Can you work these out from the model? Positions are in its coordinate system, mm. A direction names the side the tool comes from. Coordinates: 2 decimals unless noted, no trailing zeros. Order: outer loops, then holes, each group sorted by start corner. A loop starts at its lowest first (then second) coordinate and runs counter-clockwise, first axis right, second up. Notation, with made-up numbers: M 70,-11.5 L 84,-11.5 A16 ccw 84,5.5 Z; hole C 48.25,-33 d6. An arc over 180 degrees is marked long. Answer as CSV lines item,"result". Start each with the question number.
1. Will these pins go through, and if not, where does the flat tip stop? pin 1 (10 mm diameter, centred on x = 11, z = 24, fed in from +Y); pin 2 (9 mm diameter, centred on x = 10.5, y = 6, fed in from +Z); pin 3 (8 mm diameter, centred on x = 10, y = 5.5, fed in from -Z).
2. If we section it at A-A (x = 10): List the corners of the cut face in (y, z) for me, plus the area to 3 significant figures.
3. If we section it at C-C (z = 30): List the corners of the cut face in (x, y) for me.
4. I need wall thicknesses on line 1 along X through (y, z) = (-16, 30); line 2 along Y through (x, z) = (10, 2.5); line 3 along Y through (x, z) = (9.5, 39). Which ranges of each line are inside material? Lowest first, please. Write a range as from..to.
5. If we section it at D-D (x = 6.25): List the corners of the cut face in (y, z) for me.
6. If we mould it in two halves opening along Y, with no side actions, what happens to faces 1 (the face through (10, -15, 30)), 2 (the face through (20, -10, 30)), 3 (the face through (14.619, 3.585, 4.93)), 4 (the face through (10.229, 11.496, 4.93))? For each: released by +Y, released by -Y, zero draft, split by the parting line, or undercut.
7. On a 3-axis mill with a long thin cutter (end or side, diameter ignored), from which of +Z, -Z, +X, -X, +Y, -Y can I reach the whole of each face in a straight line? I mean faces 5 (the face through (10, -8, 0)), 6 (the face through (8.6, 10.5, 10)), 7 (the face through (8.418, -17.535, 32.063)). Say none if no direction works.
8. If we section it at B-B (y = 5.5): List the corners of the cut face in (x, z) for me, plus the area to 3 significant figures.
```python
from build123d import *

# Parameters (mm, degrees)
SKETCH1_W           = 20
SKETCH1_H           = 20
BOSS_EXTRUDE1_DEPTH = 60
SKETCH2_R           = 2.6
CUT_EXTRUDE1_DEPTH  = 5
SKETCH3_R           = 6
SKETCH3_R_2         = 5
BOSS_EXTRUDE2_DEPTH = 10


with BuildPart() as part:
    # Sketch1 → Boss-Extrude1 (new body)
    with BuildSketch(Plane.XY):
        with Locations((10, -10)):
            Rectangle(SKETCH1_W, SKETCH1_H)
    extrude(amount=BOSS_EXTRUDE1_DEPTH)

    # Sketch2 → Cut-Extrude1 (cut)
    with BuildSketch(Plane.XZ.offset(20)):
        with Locations(Location((10, 30, 0), (0, 0, 270))):
            Circle(SKETCH2_R)
    extrude(amount=-CUT_EXTRUDE1_DEPTH, mode=Mode.SUBTRACT)

    # Sketch3 → Boss-Extrude2 (add)
    with BuildSketch(Plane.XY):
        with Locations((10, 5.5)):
            Circle(SKETCH3_R)
        with Locations((10, 5.5)):
            Circle(SKETCH3_R_2, mode=Mode.SUBTRACT)
    extrude(amount=BOSS_EXTRUDE2_DEPTH)


solid = part.part
```
Solved:
1,pin 1,"y = 0"
1,pin 2,"z = 10"
1,pin 3,"through"
2,outline,"M -20,0 L 0.5,0 L 0.5,10 L 0,10 L 0,60 L -20,60 L -20,32.6 L -15,32.6 L -15,27.4 L -20,27.4 Z; M 10.5,0 L 11.5,0 L 11.5,10 L 10.5,10 Z"
2,area,"1,190 mm²"
3,outline,"M 0,-20 L 7.4,-20 L 7.4,-15 L 12.6,-15 L 12.6,-20 L 20,-20 L 20,0 L 0,0 Z"
4,line 1,"0..7.4, 12.6..20"
4,line 2,"-20..0.5, 10.5..11.5"
4,line 3,"-20..0"
5,outline,"M -20,0 L 0,0 L 0,60 L -20,60 Z; M 0.82,0 L 2.19,0 L 2.19,10 L 0.82,10 Z; M 8.81,0 L 10.18,0 L 10.18,10 L 8.81,10 Z"
6,face 1,"released by -Y"
6,face 2,"zero draft"
6,face 3,"undercut"
6,face 4,"undercut"
7,face 5,"-Z, +X, -X, +Y, -Y"
7,face 6,"+Z, +X, -X, +Y"
7,face 7,"-Y"
8,outline,"M 4,0 L 5,0 L 5,10 L 4,10 Z; M 15,0 L 16,0 L 16,10 L 15,10 Z"
8,area,"20.0 mm²"
